Input: part model. Units: mm. Frame: model coordinates. Face numbers are marked on the shaded views. A direction names the side the tool comes from. Give positions to 0.01 mm unless a question says otherwise; leave off trailing zeros. Loops run counter-clockwise (first coordinate to the right, second up) from the corner with the lowest first, then second, coordinate; pieces in that order, holes last. Notation, with made-up numbers: (57.5, -0.75) - (98.5, -0.75) arc R27 cw to (98.5, 17.25) - close; hole circle Ø2 at (24, -27.5). An arc over 180 degrees is marked (long way). Answer as a JSON object with one key per item and string values.
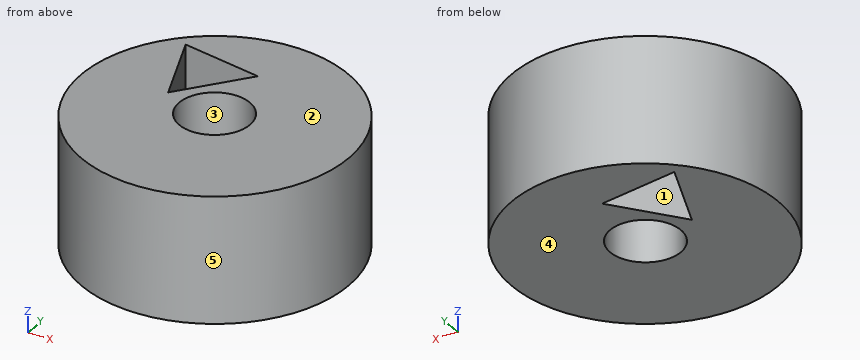
from build123d import *

# Parameters (mm, degrees)
F0_R     = 55.5167866595
F1_DEPTH = 26.2752361596
F3_DEPTH = 74.1270780563
F4_R     = 14.7193
F5_DEPTH = 121.8407154083


with BuildPart() as f1:
    # F0 (on Top) → F1 (new body, symmetric)
    with BuildSketch(Plane.XY):
        with Locations((1.0372549295, -1.4521926641)):
            Circle(F0_R)
    extrude(amount=F1_DEPTH, both=True)

    # F2 (on face) → F3 (cut)
    with BuildSketch(Plane.XY.offset(26.2752361596)):
        Polygon((-21.6351760827, 4.3129721936), (0, 30.081294477), (-33.1336097517, 35.9337454382), align=None)
    extrude(amount=-F3_DEPTH, mode=Mode.SUBTRACT)

    # F4 (on face) → F5 (cut)
    with BuildSketch(Plane.XY.offset(26.2752361596)):
        Circle(F4_R)
    extrude(amount=-F5_DEPTH, mode=Mode.SUBTRACT)


solid = f1.part
Item 1: Cut plane B-B (y = 12). Return loops of the section in (x, z).
Geometry check:
{"outline": "(-52.83, -26.28) - (-24.43, -26.28) - (-24.43, 26.28) - (-52.83, 26.28) - close; (-15.18, -26.28) - (-8.52, -26.28) - (-8.52, 26.28) - (-15.18, 26.28) - close; (8.52, -26.28) - (54.9, -26.28) - (54.9, 26.28) - (8.52, 26.28) - close"}
Item 2: Cut plane D-D (z = 15). Return loops of the section in (x, y), then the cut area to 3 significant figures.
Geometry check:
{"outline": "circle Ø111.03 at (1.04, -1.45); hole (-33.13, 35.93) - (-21.64, 4.31) - (0, 30.08) - close; hole circle Ø29.44 at (0, 0)", "area": "8,510 mm2"}
Item 3: Cut plane C-C (y = -13). Return loops of the section in (x, z).
Geometry check:
{"outline": "(-53.27, -26.28) - (-6.9, -26.28) - (-6.9, 26.28) - (-53.27, 26.28) - close; (6.9, -26.28) - (55.34, -26.28) - (55.34, 26.28) - (6.9, 26.28) - close"}
Item 4: Material intervals for line 1 (X direction, y = 20, z = 20); line 2 (X direction, y = 19, z = 5); line 3 (Y direction, x = 12.5, z = -7), sorted ascending. Write a range as [from, to].
Geometry check:
{"line 1": "x = [-50.17, -27.34], [-8.46, 52.24]", "line 2": "x = [-50.57, -26.98], [-9.3, 52.65]", "line 3": "y = [-55.77, -7.77], [7.77, 52.87]"}
Item 5: Contact query for flat-ended pins moving along their axis: P1, Ø6, axis at y = 34.5, z = 9, coming from the +X side; P2, Ø8, axis at x = 42.5, z = 12.5, coming from the -Y side; P3, Ø12, axis at y = -7, z = 2, coming from the -X side; P4, Ø4, axis at y = -6, z = 14.5, coming from the +X side. Output: stop coordinate, or through.
Geometry check:
{"P1": "stops at x = 45.72", "P2": "stops at y = -42.42", "P3": "stops at x = -54.48", "P4": "stops at x = 56.5"}
Item 6: Access query for the marked faces 1 and 2. Directions: +Z, -Z, +X, -X, +Y, -Y. A direction counts if a zero-diameter tool reaches every point of the face in a straight line with its end or side. Return the directions, or none.
Geometry check:
{"face 1": "+Z, -Z", "face 2": "+Z, +X, -X, +Y, -Y"}
Item 7: Cut plane A-A (x = -23). Return loops of the section in (y, z).
Geometry check:
{"outline": "(-51.5, -26.28) - (8.07, -26.28) - (8.07, 26.28) - (-51.5, 26.28) - close; (34.14, -26.28) - (48.59, -26.28) - (48.59, 26.28) - (34.14, 26.28) - close"}
Item 8: Mould query, pull axis Y, two halves, no side actions, for the marked faces 3, 4 and 5. Classes: released by +Y, released by -Y, zero draft, split by the parting line, or undercut.
Geometry check:
{"face 3": "undercut", "face 4": "zero draft", "face 5": "split by the parting line"}
